Design review of the part built by this model. Coordinates are the model's own, in mm. A direction names the side the tool comes from. Give positions to 0.01 mm unless a question says otherwise; leave off trailing zeros. Loops run counter-clockwise (first coordinate to the right, second up) from the corner with the lowest first, then second, coordinate; pieces in that order, holes last. Notation, with made-up numbers: (62, 81.25) -> (113, 81.25) arc R19 cw to (113, 85.25) -> close; hole circle Ø6 at (50, 9). An arc over 180 degrees is marked (long way). Use a Markdown table: item, result. Add a question column.
1. Add section C-C (z = 137). State the section outline as (x, y) points, and give its area (3 significant figures).
2. For pin 1 Ø4.5 at (y, z) = (78.5, 135) entering from +X; pin 2 Ø2 at (y, z) = (169, 161.5) entering from +X; pin 3 Ø3 at (y, z) = (83, 148) entering from -X, all flat-tipped, find the tip position at first contact; note any pin that passes through.
3. Add section B-B (x = 152.5). State the section outline as (y, z) points, and give its area (3 significant figures).
4. Add section A-A (z = 94). State the section outline as (x, y) points, and give its area (3 significant figures).
5. For faces 1 (the flat face through (167, 106, 160)), 2 (the flat face through (137.841, 84, 155)), 3 (the flat face through (200, 84, 145.3)), 4 (the flat face through (167, 167, 162.5)), 5 (the cylindrical face through (74.3, 80.12, 79.06)), list the 3-axis set-ups (+Z, -Z, +X, -X, +Y, -Y) from which the entire face can be reached by the end or side of a thin tool; tool diameter is ignored.
6. To check wall thickness, follow line 1 (X direction, y = 213, z = 135.5); line 2 (Z direction, x = 153.5, y = 219); line 3 (Y direction, x = 91, z = 82.5). State the ranges of each line that lie inside material, in increasing order.
7. Draft analysis for pull direction X (two halves, no side actions). For faces 6 (the flat face through (197.841, 85, 155)), 7 (the flat face through (167, 160, 0)), 8 (the cylindrical face through (66.46, 158.53, 3.82)), state which applies: pulls with the +X half, pulls with the -X half, needs draft (parallel to the pull), parting line crosses it, or undercut.
Autodesk Inventor part; units mm, degrees
ref_plane "YZ Plane" through (0, 0, 0) normal (1, 0, 0) x (0, 1, 0)
ref_plane "XZ Plane" through (0, 0, 0) normal (0, 1, 0) x (-1, 0, 0)
ref_plane "XY Plane" through (0, 0, 0) normal (0, 0, 1) x (1, 0, 0)
sketch "Sketch1" plane through (0, 0, 0) normal (0, 0, 1) x (1, 0, 0)
  line L0 (100.9409, 69.2591) -> (234.7409, 69.2591)
  line L1 (272.8409, 107.3591) -> (272.8409, 211.1591)
  line L2 (234.7409, 249.2591) -> (100.9409, 249.2591)
  line L3 (62.8409, 211.1591) -> (62.8409, 107.3591)
  arc A0 (100.9409, 249.2591) -> (62.8409, 211.1591) centre (100.9409, 211.1591) ccw
  arc A1 (272.8409, 211.1591) -> (234.7409, 249.2591) centre (234.7409, 211.1591) ccw
  arc A2 (234.7409, 69.2591) -> (272.8409, 107.3591) centre (234.7409, 107.3591) ccw
  arc A3 (62.8409, 107.3591) -> (100.9409, 69.2591) centre (100.9409, 107.3591) ccw
  point P0 (0, 0)
  point P1 (62.8409, 69.2591)
  point P2 (272.8409, 249.2591)
  point P3 (272.8409, 69.2591)
  dimension "d0" = 210
  dimension "d1" = 180
  dimension "d2" = 38.1
  dimension "d3" = 38.1
extrude "Extrusion1" add sketch "Sketch1" along normal blind 160
fillet "Fillet1" radius 12.7 16 edges at (261.6817, 238.0999, 0) (167.8409, 249.2591, 0) (74.0001, 238.0999, 0) (62.8409, 159.2591, 0) (74.0001, 80.4183, 0) (167.8409, 69.2591, 0) (261.6817, 80.4183, 0) (272.8409, 159.2591, 0) (261.6817, 238.0999, 160) (167.8409, 249.2591, 160) (74.0001, 238.0999, 160) (62.8409, 159.2591, 160) (74.0001, 80.4183, 160) (167.8409, 69.2591, 160) (261.6817, 80.4183, 160) (272.8409, 159.2591, 160)
sketch "Sketch2" plane through (0, 0, 160) normal (0, 0, 1) x (1, 0, 0)
  line L0 (234.7409, 69.2591) -> (100.9409, 69.2591)
  line L1 (137.8409, 99.2591) -> (197.8409, 99.2591)
  line L2 (197.8409, 99.2591) -> (197.8409, 69.2591)
  line L3 (197.8409, 69.2591) -> (137.8409, 69.2591)
  line L4 (137.8409, 69.2591) -> (137.8409, 99.2591)
  line L5 (234.7409, 81.9591) -> (100.9409, 81.9591)
  point P0 (0, 0)
  point P1 (167.8409, 99.2591)
  point P2 (167.8409, 81.9591)
  dimension "d7" = 60
  dimension "d8" = 30
extrude "Extrusion2" cut sketch "Sketch2" against normal blind 30
sketch "Sketch3" plane through (137.8409, 99.2591, 160) normal (0, -1, 0) x (1, 0, 0)
  line L0 (96.9, -12.7) -> (-36.9, -12.7)
  circle A0 centre (30, -12.7) radius 2.5
  point P0 (-137.8409, -160)
  dimension "d11" = 5
extrude "Extrusion3" add sketch "Sketch3" along normal blind 30
thread "Thread1"
sketch "Sketch4" plane through (0, 0, 160) normal (0, 0, 1) x (1, 0, 0)
  line L0 (260.1409, 107.3591) -> (260.1409, 211.1591)
  line L1 (75.5409, 211.1591) -> (260.1409, 211.1591)
  line L2 (260.1409, 211.1591) -> (260.1409, 121.1591)
  line L3 (260.1409, 121.1591) -> (75.5409, 121.1591)
  line L4 (75.5409, 121.1591) -> (75.5409, 211.1591)
  point P0 (0, 0)
  dimension "d16" = 90
extrude "Extrusion4" add sketch "Sketch4" along normal blind 2.5
sketch "Sketch5" plane through (100.9409, 69.2591, 12.7) normal (0, -1, 0) x (1, 0, 0)
  line L0 (36.9, 134.6) -> (36.9, 147.3)
  line L1 (36.9, 147.3) -> (0, 147.3)
  line L2 (0, 134.6) -> (0, 147.3)
  line L3 (0, 134.6) -> (36.9, 134.6)
  line L4 (96.9, 147.3) -> (96.9, 134.6)
  line L5 (96.9, 134.6) -> (133.8, 134.6)
  line L6 (133.8, 134.6) -> (133.8, 147.3)
  line L7 (133.8, 147.3) -> (96.9, 147.3)
  line L8 (96.9, 134.6) -> (96.9, 117.3)
  line L9 (96.9, 117.3) -> (36.9, 117.3)
  line L10 (36.9, 117.3) -> (36.9, 134.6)
  line L11 (0, 134.6) -> (36.9, 134.6)
  line L12 (0, 0) -> (0, 134.6)
  line L13 (133.8, 0) -> (0, 0)
  line L14 (133.8, 0) -> (133.8, 134.6)
  line L15 (96.9, 134.6) -> (133.8, 134.6)
  line L16 (31.9, 136.6) -> (36.9, 136.6)
  line L17 (36.9, 136.6) -> (36.9, 132.6)
  line L18 (36.9, 132.6) -> (31.9, 132.6)
  line L19 (31.9, 132.6) -> (31.9, 136.6)
  line L20 (96.9, 136.6) -> (101.9, 136.6)
  line L21 (101.9, 136.6) -> (101.9, 132.6)
  line L22 (101.9, 132.6) -> (96.9, 132.6)
  line L23 (96.9, 132.6) -> (96.9, 136.6)
  point P0 (-100.9409, -12.7)
  dimension "d19" = 4
  dimension "d20" = 5
extrude "Extrusion5" cut sketch "Sketch5" against normal blind 30 contours L3 L19 L16 L0 | L10 L18 L19 L3 | L8 L5 L21 L22 | L4 L20 L21 L5
properties part number "Robot_face"
Taken from the geometry:
| question | item | result |
|---|---|---|
| 1 | outline | (62.84, 107.36) arc R38.1 ccw to (100.94, 69.26) -> (137.84, 69.26) -> (137.84, 99.26) -> (197.84, 99.26) -> (197.84, 69.26) -> (234.74, 69.26) arc R38.1 ccw to (272.84, 107.36) -> (272.84, 211.16) arc R38.1 ccw to (234.74, 249.26) -> (100.94, 249.26) arc R38.1 ccw to (62.84, 211.16) -> close |
| 1 | area | 34,800 mm^2 |
| 2 | pin 1 | stops at x = 262.01 |
| 2 | pin 2 | stops at x = 260.14 |
| 2 | pin 3 | stops at x = 70.48 |
| 3 | outline | (69.26, 12.7) arc R12.7 ccw to (81.96, 0) -> (236.56, 0) arc R12.7 ccw to (249.26, 12.7) -> (249.26, 147.3) arc R12.7 ccw to (236.56, 160) -> (211.16, 160) -> (211.16, 162.5) -> (121.16, 162.5) -> (121.16, 160) -> (99.26, 160) -> (99.26, 130) -> (69.26, 130) -> close |
| 3 | area | 28,000 mm^2 |
| 4 | outline | (62.84, 107.36) arc R38.1 ccw to (100.94, 69.26) -> (234.74, 69.26) arc R38.1 ccw to (272.84, 107.36) -> (272.84, 211.16) arc R38.1 ccw to (234.74, 249.26) -> (100.94, 249.26) arc R38.1 ccw to (62.84, 211.16) -> close |
| 4 | area | 36,600 mm^2 |
| 5 | face 1 | +Z, +X, -X, -Y |
| 5 | face 2 | +Z, -Y |
| 5 | face 3 | -Y |
| 5 | face 4 | +Z, +X, -X, +Y, -Y |
| 5 | face 5 | +Z, -Z, -X, -Y |
| 6 | line 1 | x = 62.89 to 272.8 |
| 6 | line 2 | z = 0 to 160 |
| 6 | line 3 | y = 70.58 to 247.94 |
| 7 | face 6 | undercut |
| 7 | face 7 | needs draft |
| 7 | face 8 | pulls with the -X half |
